Verification items for the finished model (mm, model axes). A direction names the side the tool comes from. Coordinates: 2 decimals unless noted, no trailing zeros. Order: outer loops, then holes, each group sorted by start corner. A loop starts at its lowest first (then second) coordinate and runs counter-clockwise, first axis right, second up. Notation, with made-up numbers: M 8,-19.75 L 22,-19.75 A13 cw 22,-4.75 Z; hole C 55.5,22.5 d10. An arc over 180 degrees is marked long. Answer as a JSON object with one key per item and string values. Group by question number.
(1) Gauge pin test, flat ends, axial feed: pin 1 Ø8 at (x, y) = (15.5, -8) entering from +Z; pin 2 Ø6 at (x, y) = (5.5, 1) entering from +Z. Record the tip position at first contact, or that the pin passes through.
(2) Cross-section at C-C (z = 8.5). Enter the section's corners in (x, y), plus the area to 3 significant figures.
(3) Material ranges on line 1 (Z direction, x = -22, y = 0); line 2 (X direction, y = -5, z = 59), recorded low to high.
(4) Mould release check, pull along Y, two halves, no side actions. Record for faces 1 (the face through (20, 0, 46)), 2 (the face through (0, -16.35, 43)), 3 (the face through (0, 0, 6.35)), 4 (the face through (0, 0, 0)): released by +Y, released by -Y, zero draft, split by the parting line, or undercut.
(5) Cross-section at B-B (x = -10.5). Enter the section's corners in (y, z), plus the area to 3 significant figures.
(6) Access from +Z, -Z, +X, -X, +Y, -Y to the whole of each face (thin tool, end or side, straight path). Record for faces 5 (the face through (26.35, 0, 43)), 6 (the face through (0, -10, 46)).
(7) Cross-section at A-A (y = 7.5). Enter the section's corners in (x, z).
from build123d import *

# Parameters (mm, degrees)
F0_W     = 52.7
F0_H     = 32.7
F1_DEPTH = 86.35
F2_T     = -6.35
F4_D     = 1
F5_D     = 1


with BuildPart() as f1:
    # F0 (on Top) → F1 (new body)
    with BuildSketch(Plane.XY):
        Rectangle(F0_W, F0_H)
    extrude(amount=F1_DEPTH)

    # F2
    f2_openings = [f1.faces().sort_by_distance(p)[0] for p in [
        (0, 0, 86.35),
    ]]
    offset(amount=F2_T, openings=f2_openings)

    # F4 (through all)
    with Locations(Plane(origin=(-26.35, 0, 0), x_dir=(0, -1, 0), z_dir=(-1, 0, 0))):
        with Locations((0, 70)):
            Hole(F4_D / 2)

    # F5 (through all)
    with Locations(Plane(origin=(-26.35, 0, 0), x_dir=(0, -1, 0), z_dir=(-1, 0, 0))):
        with Locations((0, 16.35)):
            Hole(F5_D / 2)


solid = f1.part
Taken from the geometry:
{
 "1": {"pin 1": "stops at z = 86.35", "pin 2": "stops at z = 6.35"},
 "2": {"outline": "M -26.35,-16.35 L 26.35,-16.35 L 26.35,16.35 L -26.35,16.35 Z; hole M -20,-10 L 20,-10 L 20,10 L -20,10 Z", "area": "923 mm²"},
 "3": {"line 1": "z = 0 to 15.85, 16.85 to 69.5, 70.5 to 86.35", "line 2": "x = -26.35 to -20, 20 to 26.35"},
 "4": {"face 1": "undercut", "face 2": "released by -Y", "face 3": "undercut", "face 4": "zero draft"},
 "5": {"outline": "M -16.35,0 L 16.35,0 L 16.35,86.35 L 10,86.35 L 10,6.35 L -10,6.35 L -10,86.35 L -16.35,86.35 Z", "area": "1,220 mm²"},
 "6": {"face 5": "+Z, -Z, +X, +Y, -Y", "face 6": "+Z"},
 "7": {"outline": "M -26.35,0 L 26.35,0 L 26.35,86.35 L 20,86.35 L 20,6.35 L -20,6.35 L -20,86.35 L -26.35,86.35 Z"}
}
